Source: CAD feature listing. Evaluate the final solid. Frame: model axes, mm. A direction names the side the tool comes from. Give positions to 0.01 mm unless a question says otherwise; leave off trailing zeros. Order: outer loops, then holes, each group sorted by start corner. A loop starts at its lowest first (then second) coordinate and runs counter-clockwise, first axis right, second up. Notation, with made-up numbers: (14.5, -7) - (29.5, -7) arc R22 cw to (29.5, 26) - close; hole circle Ø1 at (52.5, -6.75). An arc over 180 degrees is marked (long way). Write each question's results on one line, items separated by ' | '. Start each with the question number.
Item 1: Mould query, pull axis X, two halves, no side actions, for faces 4 (the flat face through (3, 2, 0)), 5 (the flat face through (0, 3.556, 0)), 6 (the flat face through (1.3, 4.064, -1.4)). Classes: released by +X, released by -X, zero draft, split by the parting line, or undercut.
Item 2: Section B-B on z = 0. Output: boundary loops of the cut face in (x, y), and give its area (3 significant figures).
Item 3: Section C-C on x = 0. Output: boundary loops of the cut face in (y, z).
Item 4: Set-up query: faces 1 (the flat face through (-3, 2, 0)), 2 (the cylindrical face through (1.73, 3.81, -0.23)), 3 (the flat face through (-2.289, -1.03, -3.17)). Return all of +Z, -Z, +X, -X, +Y, -Y with unobstructed straight access to the full face (end or side cutting, diameter ignored); none if empty.
Item 5: Contact query for flat-ended pins moving along their axis: pin 1 Ø1.5 at (x, y) = (0.5, 0) entering from -Z; pin 2 Ø2 at (x, y) = (-2, 1.5) entering from +Z; pin 3 Ø3 at (x, z) = (1.5, 1) entering from -Y. Output: stop coordinate, or through.
Item 6: Section A-A on y = -1.25. Output: boundary loops of the cut face in (x, z).
Item 7: Line query: line 1 along X through (y, z) = (3.8, 0); line 2 along Z through (x, y) = (-2.5, -1.5); line 3 along Z through (x, y) = (0, 3.25). Output: solid intervals per line, ascending.
Item 8: Section D-D on y = 3. Output: boundary loops of the cut face in (x, z), and give its area (3 significant figures).
```python
from build123d import *

# Parameters (mm, degrees)
SKETCH1_W            = 6
SKETCH1_H            = 6
BOSS_EXTRUDE1_DEPTH  = 4.064
BOSS_EXTRUDE2_DEPTH  = 0.7112
LPATTERN1_COUNT      = 2
LPATTERN1_PITCH      = 5.288799938
MIRROR1_COPY_1_DEPTH = 0.7112
SKETCH3_R            = 1.74625
CUT_EXTRUDE1_DEPTH   = 0.508


with BuildPart() as part:
    # Sketch1 → Boss-Extrude1 (new body)
    with BuildSketch(Plane(origin=(0, 0, 0), x_dir=(1, 0, 0), z_dir=(0, 1, 0))):
        Rectangle(SKETCH1_W, SKETCH1_H)
    extrude(amount=BOSS_EXTRUDE1_DEPTH)

    # Sketch2 → Boss-Extrude2 (add)
    with BuildSketch(Plane(origin=(3, 0, 0), x_dir=(0, 0, -1), z_dir=(1, 0, 0))):
        Polygon((-3, 0), (-3, -1.524), (-2.381416261, -2.633168228), (-2.6698, -2.794), (-3.3302, -1.609852), (-3.3302, 0.508), (-3, 0.508), align=None)
    boss_extrude2 = extrude(amount=-BOSS_EXTRUDE2_DEPTH)

    # LPattern1: Boss-Extrude2 ×2
    with Locations(*[(-i * LPATTERN1_PITCH, 0, 0) for i in range(1, LPATTERN1_COUNT)]):
        add(boss_extrude2)

    # Mirror1: Boss-Extrude2 across plane
    add(boss_extrude2.mirror(Plane.XY))

    # Mirror1 copy 1 sketch → Mirror1 copy 1 (add)
    with BuildSketch(Plane(origin=(-2.288799938, 0, 0), x_dir=(0, 0, 1), z_dir=(1, 0, 0))):
        Polygon((-3, 0), (-3, 1.524), (-2.381416261, 2.633168228), (-2.6698, 2.794), (-3.3302, 1.609852), (-3.3302, -0.508), (-3, -0.508), align=None)
    extrude(amount=-MIRROR1_COPY_1_DEPTH)

    # Sketch3 → Cut-Extrude1 (cut)
    with BuildSketch(Plane(origin=(0, 4.064, 0), x_dir=(1, 0, 0), z_dir=(0, 1, 0))):
        with Locations(Location((0, 0, 0), (0, 0, 270))):
            Circle(SKETCH3_R)
    extrude(amount=-CUT_EXTRUDE1_DEPTH, mode=Mode.SUBTRACT)


solid = part.part
```
Evaluation:
1) face 4: released by +X | face 5: undercut | face 6: zero draft
2) outline: (-3, 0) - (3, 0) - (3, 4.06) - (1.75, 4.06) - (1.75, 3.56) - (-1.75, 3.56) - (-1.75, 4.06) - (-3, 4.06) - close | area: 22.6 mm^2
3) outline: (0, -3) - (4.06, -3) - (4.06, -1.75) - (3.56, -1.75) - (3.56, 1.75) - (4.06, 1.75) - (4.06, 3) - (0, 3) - close
4) face 1: +Z, -Z, -X, +Y, -Y | face 2: +Y | face 3: -Z, -Y
5) pin 1: stops at z = -3 | pin 2: stops at z = 3 | pin 3: stops at y = 0
6) outline: (-3, -3.33) - (-2.29, -3.33) - (-2.29, -3) - (-3, -3) - close; (-3, 3) - (-2.29, 3) - (-2.29, 3.33) - (-3, 3.33) - close; (2.29, -3.33) - (3, -3.33) - (3, -3) - (2.29, -3) - close; (2.29, 3) - (3, 3) - (3, 3.33) - (2.29, 3.33) - close
7) line 1: x = -3 to -1.75, 1.75 to 3 | line 2: z = -3.33 to -3, 3 to 3.33 | line 3: z = -3 to 3
8) outline: (-3, -3) - (3, -3) - (3, 3) - (-3, 3) - close | area: 36.0 mm^2
